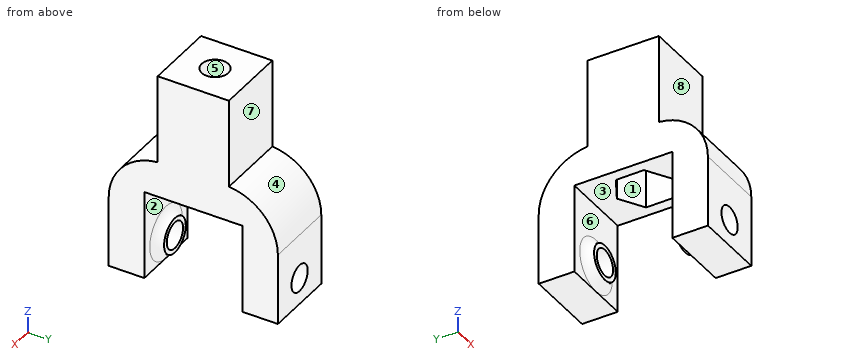
from build123d import *

# Parameters (mm, degrees)
EXTRUDE_1_DEPTH     = 8
CUT_EXTRUDE_1_REACH = 26.92
SKETCH_4_R          = 1.5
EXTRUDE_START       = 1
SKETCH_5_R          = 2
SKETCH_5_R_2        = 1.5
EXTRUDE_2_DEPTH     = 1
SKETCH_6_R          = 2
SKETCH_6_R_2        = 1.5
EXTRUDE_3_DEPTH     = 1
FILLET_1_R          = 1
FILLET_2_R          = 1
SKETCH_10_W         = 8
SKETCH_10_H         = 8
EXTRUDE_5_DEPTH     = 10
SKETCH_7_R          = 1.5
CUT_EXTRUDE_2_DEPTH = 14
CUT_EXTRUDE_3_DEPTH = 10
FILLET_3_R          = 6
FILLET_4_R          = 6


# Some blends are built 0.0001 mm under size
with BuildPart() as part:
    # Эскиз3 → Бобышка-Вытянуть1 (new body)
    with BuildSketch(Plane(origin=(0, 0, 0), x_dir=(0, 0, -1), z_dir=(1, 0, 0))):
        Polygon((0, 0), (14, 0), (14, 4), (4, 4), (4, 15), (14, 15), (14, 19), (0, 19), align=None)
    extrude(amount=EXTRUDE_1_DEPTH)

    # Вырез-Вытянуть1: up to this face of the body (flat: up to its plane)
    cut_extrude_1_end = Plane(part.part.faces().sort_by_distance((4, 0, -7))[0])
    # Эскиз4 → Вырез-Вытянуть1 (cut, up to the picked face)
    with BuildSketch(Plane(origin=(0, 19, 0), x_dir=(1, 0, 0), z_dir=(0, 1, 0)), mode=Mode.PRIVATE) as cut_extrude_1_sk1:
        with Locations(Location((4, 11, 0), (0, 0, 270))):
            Circle(SKETCH_4_R)
    cut_extrude_1_tool1 = split(extrude(cut_extrude_1_sk1.sketch, amount=-CUT_EXTRUDE_1_REACH, mode=Mode.PRIVATE), bisect_by=cut_extrude_1_end, keep=Keep.BOTH, mode=Mode.PRIVATE)
    add(cut_extrude_1_tool1.solids().sort_by(Axis((4, 19, -11), (0, -1, 0)))[0], mode=Mode.SUBTRACT)

    # Эскиз5 → Бобышка-Вытянуть2 (add)
    with BuildSketch(Plane(origin=(0, 4, 0), x_dir=(1, 0, 0), z_dir=(0, 1, 0)).offset(EXTRUDE_START)):
        with Locations(Location((4, 11, 0), (0, 0, 90))):
            Circle(SKETCH_5_R)
        with Locations(Location((4, 11, 0), (0, 0, 270))):
            Circle(SKETCH_5_R_2, mode=Mode.SUBTRACT)
    extrude(amount=-EXTRUDE_2_DEPTH)

    # Эскиз6 → Бобышка-Вытянуть3 (add)
    with BuildSketch(Plane(origin=(0, 15, 0), x_dir=(-1, 0, 0), z_dir=(0, -1, 0))):
        with Locations(Location((-4, 11, 0), (0, 0, 90))):
            Circle(SKETCH_6_R)
        with Locations(Location((-4, 11, 0), (0, 0, 270))):
            Circle(SKETCH_6_R_2, mode=Mode.SUBTRACT)
    extrude(amount=EXTRUDE_3_DEPTH)

    # Скругление1
    fillet_1_edges = [part.edges().sort_by_distance(p)[0] for p in [
        (4, 4, -9),
    ]]
    fillet(fillet_1_edges, radius=FILLET_1_R - 0.0001)  # a hair under: the kernel refuses the full size

    # Скругление2
    fillet_2_edges = [part.edges().sort_by_distance(p)[0] for p in [
        (4, 15, -9),
    ]]
    fillet(fillet_2_edges, radius=FILLET_2_R - 0.0001)  # a hair under: the kernel refuses the full size

    # Эскиз10 → Бобышка-Вытянуть5 (add)
    with BuildSketch(Plane.XY):
        with Locations((4, 9.5)):
            Rectangle(SKETCH_10_W, SKETCH_10_H)
    extrude(amount=EXTRUDE_5_DEPTH)

    # Эскиз7 → Вырез-Вытянуть2 (cut)
    with BuildSketch(Plane(origin=(0, 0, -4), x_dir=(-1, 0, 0), z_dir=(0, 0, -1))):
        with Locations((-4, 9.5)):
            Circle(SKETCH_7_R)
    extrude(amount=-CUT_EXTRUDE_2_DEPTH, mode=Mode.SUBTRACT)

    # Эскиз9 → Вырез-Вытянуть3 (cut)
    with BuildSketch(Plane(origin=(0, 0, -4), x_dir=(-1, 0, 0), z_dir=(0, 0, -1))):
        Polygon((-1.264118223, 11.111919426), (-4.028022284, 12.675302834), (-6.763904061, 11.063383407), (-6.735881777, 7.888080574), (-3.971977716, 6.324697166), (-1.236095939, 7.936616593), align=None)
    extrude(amount=-CUT_EXTRUDE_3_DEPTH, mode=Mode.SUBTRACT)

    # Скругление3
    # the kernel refuses this fillet: 6 mm, written as the material it takes off along each edge
    with BuildSketch(Plane(origin=(-14.947825929, 19, 0), x_dir=(0, 0, -1), z_dir=(1, 0, 0))) as fillet_3_piece_1:
        with BuildLine():
            CenterArc((5.979130372, -6), FILLET_3_R, 90, 85.219808153)
            Line((0, -5.5), (-0.119582607, -5.49))
            ThreePointArc((-0.119582607, -5.49), (-0.12, -2.75), (-0.12, 0))
            Line((-0.12, 0), (0, 0.12))
            Line((0, 0.12), (5.979130372, 0.12))
            Line((5.979130372, 0.12), (5.979130372, 0))
        make_face()
    extrude(amount=37.895651858, mode=Mode.SUBTRACT)

    # Скругление4
    # the kernel refuses this fillet: 6 mm, written as the material it takes off along each edge
    with BuildSketch(Plane(origin=(-14.947825929, 0, 0), x_dir=(0, 1, 0), z_dir=(1, 0, 0))) as fillet_4_piece_1:
        with BuildLine():
            CenterArc((6, -5.979130372), FILLET_4_R, 94.780191847, 85.219808153)
            Line((0, -5.979130372), (-0.12, -5.979130372))
            Line((-0.12, -5.979130372), (-0.12, 0))
            Line((-0.12, 0), (0, 0.12))
            ThreePointArc((0, 0.12), (2.75, 0.12), (5.49, 0.119582607))
            Line((5.49, 0.119582607), (5.5, 0))
        make_face()
    extrude(amount=37.895651858, mode=Mode.SUBTRACT)


solid = part.part
Model file for the job. Use its own axes, mm. Face numbers are marked on the shaded views. A direction names the side the tool comes from. Give positions to 0.01 mm unless a question says otherwise; leave off trailing zeros. Loops run counter-clockwise (first coordinate to the right, second up) from the corner with the lowest first, then second, coordinate; pieces in that order, holes last. Notation, with made-up numbers: (65.25, 35) - (91.25, 35) arc R19 cw to (91.25, 40) - close; hole circle Ø9 at (62.5, 67.25). An arc over 180 degrees is marked (long way). Use one line per item in the form item = value.
(1) Drill centre lines: L1, parallel to X at y = 17, z = -11; L2, parallel to Y at x = 4, z = 8.45; L3, parallel to X at y = 18, z = -10.5. Where is each one in solid material? Low to high.
Determined:
L1 = 0 to 2.5, 5.5 to 8
L2 = 5.5 to 8, 11 to 13.5
L3 = 0 to 2.59, 5.41 to 8
(2) Pull direction Y, two halves, no side cores. Call the marked faces 5, 6, 7 and 8: pulls with the +Y half, pulls with the -Y half, needs draft (parallel to the pull), parting line crosses it, or undercut.
Determined:
face_5 = undercut
face_6 = undercut
face_7 = pulls with the +Y half
face_8 = pulls with the -Y half
(3) Cut at D-D (z = 7.5). Give the cut face in (x, y).
Determined:
outline = (0, 5.5) - (8, 5.5) - (8, 13.5) - (0, 13.5) - close; hole circle Ø3 at (4, 9.5)
(4) 3-axis set-ups, long thin cutter, end or side, ignore diameter. For the marked faces 1, 2, 3 and 4: which of +Z, -Z, +X, -X, +Y, -Y reach the whole face in a straight line?
Determined:
face_1 = -Z
face_2 = none
face_3 = +X, -X
face_4 = +Z, +X, -X, +Y
(5) Cut at B-B (y = 9.5). Give the cut face in (x, z), then the cut area to 3 significant figures.
Determined:
outline = (0, -4) - (1.25, -4) - (1.25, 6) - (2.5, 6) - (2.5, 10) - (0, 10) - close; (5.5, 6) - (6.75, 6) - (6.75, -4) - (8, -4) - (8, 10) - (5.5, 10) - close
area = 45.0 mm^2
(6) Cut at A-A (z = -11). Count the separate pieces of the cut face and the enclosed holes in it, then the cut area to 3 significant figures.
Determined:
separate_pieces = 4
enclosed_holes = 0
area = 42.9 mm^2
(7) Cut at C-C (y = 14.5). Give the cut face in (x, z).
Determined:
outline = (0, -4) - (8, -4) - (8, -0.17) - (0, -0.17) - close; circle Ø4.27 at (4, -11); hole circle Ø3 at (4, -11)
(8) Drop flat-ended pins along their axis: P1, Ø10, axis at y = 2.5, z = -1, coming from the -X side; P2, Ø2.5, axis at x = 4.5, z = 5.5, coming from the +Y side; P3, Ø2.5, axis at x = 4, z = -11, coming from the +Y side; P4, Ø2.5, axis at x = 3, z = 4.5, coming from the -Y side. Give the stop position or say it passes through.
Determined:
P1 = 0
P2 = 13.5
P3 = through
P4 = 5.5
